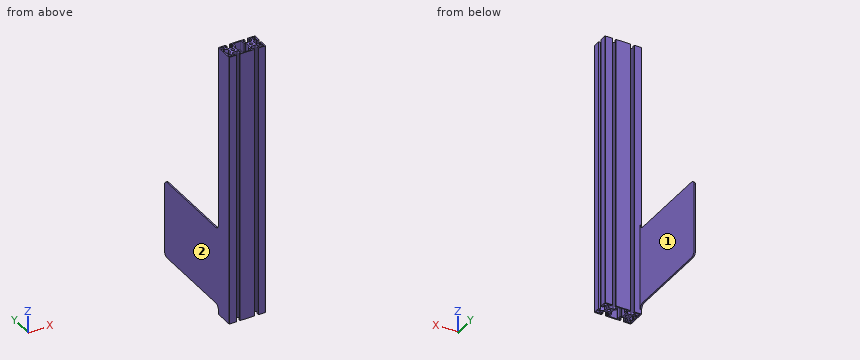
from build123d import *

# Parameters (mm, degrees)
SZKIC1_R                    = 3.4
DODANIE_WYCI_GNI_CIE1_DEPTH = 600
SZKIC2_W                    = 170
SZKIC2_H                    = 200
DODANIE_WYCI_GNI_CIE3_DEPTH = 3
ZAOKR_GLENIE1_R             = 10


with BuildPart() as part:
    # Szkic1 → Dodanie-wyciągnięcie1 (new body)
    with BuildSketch(Plane.XY):
        with BuildLine():
            Line((-40, -19), (-40, 20))
            Line((-40, 20), (-24, 20))
            Line((-24, 20), (-24, 15.5))
            Line((-24, 15.5), (-26.471381771, 15.5))
            Line((-26.471381771, 15.5), (-26.471381771, 17.75))
            ThreePointArc((-26.471381771, 17.75), (-28.062372029, 17.090990258), (-28.721381771, 15.5))
            ThreePointArc((-28.721381771, 15.5), (-27.448087912, 10.962546258), (-24, 7.75))
            Line((-24, 7.75), (-16, 7.75))
            ThreePointArc((-16, 7.75), (-12.551912088, 10.962546258), (-11.278618229, 15.5))
            ThreePointArc((-11.278618229, 15.5), (-11.937627971, 17.090990258), (-13.528618229, 17.75))
            Line((-13.528618229, 17.75), (-13.528618229, 15.5))
            Line((-13.528618229, 15.5), (-16, 15.5))
            Line((-16, 15.5), (-16, 20))
            Line((-16, 20), (13.528618229, 20))
            Line((13.528618229, 20), (16, 20))
            Line((16, 20), (16, 15.5))
            Line((16, 15.5), (13.528618229, 15.5))
            Line((13.528618229, 15.5), (13.528618229, 17.75))
            ThreePointArc((13.528618229, 17.75), (11.937627971, 17.090990258), (11.278618229, 15.5))
            ThreePointArc((11.278618229, 15.5), (12.551912088, 10.962546258), (16, 7.75))
            Line((16, 7.75), (24, 7.75))
            ThreePointArc((24, 7.75), (27.448087912, 10.962546258), (28.721381771, 15.5))
            ThreePointArc((28.721381771, 15.5), (28.062372029, 17.090990258), (26.471381771, 17.75))
            Line((26.471381771, 17.75), (26.471381771, 15.5))
            Line((26.471381771, 15.5), (24, 15.5))
            Line((24, 15.5), (24, 20))
            Line((24, 20), (39, 20))
            ThreePointArc((39, 20), (39.707106781, 19.707106781), (40, 19))
            Line((40, 19), (40, 4))
            Line((40, 4), (35.5, 4))
            Line((35.5, 4), (35.5, 6.471381771))
            Line((35.5, 6.471381771), (37.75, 6.471381771))
            ThreePointArc((37.75, 6.471381771), (37.090990258, 8.062372029), (35.5, 8.721381771))
            ThreePointArc((35.5, 8.721381771), (30.962546258, 7.448087912), (27.75, 4))
            Line((27.75, 4), (27.75, -4))
            ThreePointArc((27.75, -4), (30.962546258, -7.448087912), (35.5, -8.721381771))
            ThreePointArc((35.5, -8.721381771), (37.090990258, -8.062372029), (37.75, -6.471381771))
            Line((37.75, -6.471381771), (35.5, -6.471381771))
            Line((35.5, -6.471381771), (35.5, -4))
            Line((35.5, -4), (40, -4))
            Line((40, -4), (40, -19))
            ThreePointArc((40, -19), (39.707106781, -19.707106781), (39, -20))
            Line((39, -20), (24, -20))
            Line((24, -20), (24, -15.5))
            Line((24, -15.5), (26.471381771, -15.5))
            Line((26.471381771, -15.5), (26.471381771, -17.75))
            ThreePointArc((26.471381771, -17.75), (28.062372029, -17.090990258), (28.721381771, -15.5))
            ThreePointArc((28.721381771, -15.5), (27.448087912, -10.962546258), (24, -7.75))
            Line((24, -7.75), (16, -7.75))
            ThreePointArc((16, -7.75), (12.551912088, -10.962546258), (11.278618229, -15.5))
            ThreePointArc((11.278618229, -15.5), (11.937627971, -17.090990258), (13.528618229, -17.75))
            Line((13.528618229, -17.75), (13.528618229, -15.5))
            Line((13.528618229, -15.5), (16, -15.5))
            Line((16, -15.5), (16, -20))
            Line((16, -20), (-16, -20))
            Line((-16, -20), (-16, -15.5))
            Line((-16, -15.5), (-13.528618229, -15.5))
            Line((-13.528618229, -15.5), (-13.528618229, -17.75))
            ThreePointArc((-13.528618229, -17.75), (-11.937627971, -17.090990258), (-11.278618229, -15.5))
            ThreePointArc((-11.278618229, -15.5), (-12.551912088, -10.962546258), (-16, -7.75))
            Line((-16, -7.75), (-24, -7.75))
            ThreePointArc((-24, -7.75), (-27.448087912, -10.962546258), (-28.721381771, -15.5))
            ThreePointArc((-28.721381771, -15.5), (-28.062372029, -17.090990258), (-26.471381771, -17.75))
            Line((-26.471381771, -17.75), (-26.471381771, -15.5))
            Line((-26.471381771, -15.5), (-24, -15.5))
            Line((-24, -15.5), (-24, -20))
            Line((-24, -20), (-39, -20))
            ThreePointArc((-39, -20), (-39.707106781, -19.707106781), (-40, -19))
        make_face()
        with Locations((-20, 0)):
            Circle(SZKIC1_R, mode=Mode.SUBTRACT)
        with Locations((20, 0)):
            Circle(SZKIC1_R, mode=Mode.SUBTRACT)
        with BuildLine():
            Line((30.971381771, -17.75), (36.75, -17.75))
            ThreePointArc((36.75, -17.75), (37.457106781, -17.457106781), (37.75, -16.75))
            Line((37.75, -16.75), (37.75, -10.971381771))
            Line((37.75, -10.971381771), (30.971381771, -10.971381771))
            Line((30.971381771, -10.971381771), (30.971381771, -17.75))
        make_face(mode=Mode.SUBTRACT)
        with BuildLine():
            Line((-35.5, -6.471381771), (-37.75, -6.471381771))
            ThreePointArc((-37.75, -6.471381771), (-37.090990258, -8.062372029), (-35.5, -8.721381771))
            ThreePointArc((-35.5, -8.721381771), (-30.962546258, -7.448087912), (-27.75, -4))
            Line((-27.75, -4), (-27.75, 4))
            ThreePointArc((-27.75, 4), (-30.962546258, 7.448087912), (-35.5, 8.721381771))
            ThreePointArc((-35.5, 8.721381771), (-37.090990258, 8.062372029), (-37.75, 6.471381771))
            Line((-37.75, 6.471381771), (-35.5, 6.471381771))
            Line((-35.5, 6.471381771), (-35.5, 4))
            Line((-35.5, 4), (-37.75, 4))
            Line((-37.75, 4), (-37.75, -4))
            Line((-37.75, -4), (-35.5, -4))
            Line((-35.5, -4), (-35.5, -6.471381771))
        make_face(mode=Mode.SUBTRACT)
        with BuildLine():
            Line((10.528618229, 7.090188806), (11.40950808, 7.090188806))
            ThreePointArc((11.40950808, 7.090188806), (12.470168251, 6.650848977), (12.90950808, 5.590188806))
            Line((12.90950808, 5.590188806), (12.90950808, -5.590188806))
            ThreePointArc((12.90950808, -5.590188806), (12.470168251, -6.650848977), (11.40950808, -7.090188806))
            Line((11.40950808, -7.090188806), (10.528618229, -7.090188806))
            ThreePointArc((10.528618229, -7.090188806), (9.467958057, -7.529528634), (9.028618229, -8.590188806))
            Line((9.028618229, -8.590188806), (9.028618229, -16.25))
            ThreePointArc((9.028618229, -16.25), (8.589278401, -17.310660172), (7.528618229, -17.75))
            Line((7.528618229, -17.75), (-7.528618229, -17.75))
            ThreePointArc((-7.528618229, -17.75), (-8.589278401, -17.310660172), (-9.028618229, -16.25))
            Line((-9.028618229, -16.25), (-9.028618229, -8.590188806))
            ThreePointArc((-9.028618229, -8.590188806), (-9.467958057, -7.529528634), (-10.528618229, -7.090188806))
            Line((-10.528618229, -7.090188806), (-11.40950808, -7.090188806))
            ThreePointArc((-11.40950808, -7.090188806), (-12.470168251, -6.650848977), (-12.90950808, -5.590188806))
            Line((-12.90950808, -5.590188806), (-12.90950808, 5.590188806))
            ThreePointArc((-12.90950808, 5.590188806), (-12.470168251, 6.650848977), (-11.40950808, 7.090188806))
            Line((-11.40950808, 7.090188806), (-10.528618229, 7.090188806))
            ThreePointArc((-10.528618229, 7.090188806), (-9.467958057, 7.529528634), (-9.028618229, 8.590188806))
            Line((-9.028618229, 8.590188806), (-9.028618229, 16.25))
            ThreePointArc((-9.028618229, 16.25), (-8.589278401, 17.310660172), (-7.528618229, 17.75))
            Line((-7.528618229, 17.75), (7.528618229, 17.75))
            ThreePointArc((7.528618229, 17.75), (8.589278401, 17.310660172), (9.028618229, 16.25))
            Line((9.028618229, 16.25), (9.028618229, 8.590188806))
            ThreePointArc((9.028618229, 8.590188806), (9.467958057, 7.529528634), (10.528618229, 7.090188806))
        make_face(mode=Mode.SUBTRACT)
        with BuildLine():
            Line((30.971381771, 10.971381771), (37.75, 10.971381771))
            Line((37.75, 10.971381771), (37.75, 16.75))
            ThreePointArc((37.75, 16.75), (37.457106781, 17.457106781), (36.75, 17.75))
            Line((36.75, 17.75), (30.971381771, 17.75))
            Line((30.971381771, 17.75), (30.971381771, 10.971381771))
        make_face(mode=Mode.SUBTRACT)
        with BuildLine():
            Line((-30.971381771, -10.971381771), (-30.971381771, -17.75))
            Line((-30.971381771, -17.75), (-36.75, -17.75))
            ThreePointArc((-36.75, -17.75), (-37.457106781, -17.457106781), (-37.75, -16.75))
            Line((-37.75, -16.75), (-37.75, -10.971381771))
            Line((-37.75, -10.971381771), (-30.971381771, -10.971381771))
        make_face(mode=Mode.SUBTRACT)
        with BuildLine():
            Line((-30.971381771, 17.75), (-36.75, 17.75))
            ThreePointArc((-36.75, 17.75), (-37.457106781, 17.457106781), (-37.75, 16.75))
            Line((-37.75, 16.75), (-37.75, 10.971381771))
            Line((-37.75, 10.971381771), (-30.971381771, 10.971381771))
            Line((-30.971381771, 10.971381771), (-30.971381771, 17.75))
        make_face(mode=Mode.SUBTRACT)
    extrude(amount=DODANIE_WYCI_GNI_CIE1_DEPTH)

    # Szkic2 → Dodanie-wyciągnięcie3 (add)
    with BuildSketch(Plane.ZY.offset(40)):
        with Locations((105, 120)):
            Rectangle(SZKIC2_W, SZKIC2_H)
    extrude(amount=-DODANIE_WYCI_GNI_CIE3_DEPTH)

    # Zaokrąglenie1
    zaokr_glenie1_edges = [part.edges().sort_by_distance(p)[0] for p in [
        (-38.5, 20, 20),
        (-38.5, 220, 20),
        (-38.5, 220, 190),
        (-38.5, 20, 190),
    ]]
    fillet(zaokr_glenie1_edges, radius=ZAOKR_GLENIE1_R)


solid = part.part
Check sheet for the modelled part. Datum: model origin and axes. Units: mm. Face numbers are marked on the shaded views. A direction names the side the tool comes from. Round coordinates to 2 decimals unless told otherwise and drop trailing zeros. Order: outer loops, then holes, each group sorted by start corner. A loop starts at its lowest first (then second) coordinate and runs counter-clockwise, first axis right, second up.
(1) Scan lines: probe 1 along Y at (x, z) = (-34, 263.5); probe 2 along X at (y, z) = (18.5, 430.5); probe 3 along X at (y, z) = (-1.5, 501). Record each from-to range of solid material in increasing order.
(2) Access from +Z, -Z, +X, -X, +Y, -Y to the whole of each face (thin tool, end or side, straight path). Record for the marked faces 1 and 2.
(3) Cross-section at B-B, the plane y = 145. Enter the section's corners in (x, z), and give its area (3 significant figures).
(4) Cross-section at A-A, the plane z = 510. State how many separate pieces and enclosed holes the cut face has, and give its area (3 significant figures).
(5) Go/stop test with flat-tipped pins: P1, Ø2, axis at x = 25, z = 446.5, coming from the +Y side; P2, Ø2.5, axis at y = 0, z = 356.5, coming from the +X side; P3, Ø6, axis at x = 20, y = 0, coming from the +Z side. Record where each tip stops, or that it passes through.
Check sheet entries:
1. probe 1: y = -20 to -17.75, -10.97 to -8.59, 8.59 to 10.97, 17.75 to 20
1. probe 2: x = -40 to -24, -16 to 16, 24 to 40
1. probe 3: x = -40 to -37.75, -27.75 to -23.05, -16.95 to -12.91, 12.91 to 16.95, 23.05 to 27.75
2. face 1: +Z, -Z, +X, +Y
2. face 2: +Z, -Z, -X, +Y, -Y
3. outline: (-40, 20) - (-37, 20) - (-37, 190) - (-40, 190) - close
3. area: 510 mm2
4. separate pieces: 1
4. enclosed holes: 8
4. area: 1,260 mm2
5. P1: stops at y = 20
5. P2: stops at x = 27.75
5. P3: passes through
